```python
from build123d import *

# Parameters (mm, degrees)
BOSS_EXTRUDE3_DEPTH = 90
SKETCH3_W           = 60
SKETCH3_H           = 60
BOSS_EXTRUDE4_DEPTH = 10
BOSS_EXTRUDE5_DEPTH = 24
CUT_EXTRUDE1_REACH  = 101.499
SKETCH6_R           = 2
CUT_EXTRUDE2_REACH  = 101.499
SKETCH7_R           = 2
CUT_EXTRUDE3_REACH  = 101.499
SKETCH9_R           = 2
CUT_EXTRUDE4_REACH  = 101.499
SKETCH10_R          = 2


with BuildPart() as part:
    # Sketch1 → Boss-Extrude3 (new body)
    with BuildSketch(Plane(origin=(0, 0, 0), x_dir=(1, 0, 0), z_dir=(0, 1, 0))):
        with BuildLine():
            Line((-20, 30), (20, 30))
            ThreePointArc((20, 30), (22.928932188, 22.928932188), (30, 20))
            Line((30, 20), (30, -20))
            ThreePointArc((30, -20), (22.928932188, -22.928932188), (20, -30))
            Line((20, -30), (-20, -30))
            ThreePointArc((-20, -30), (-22.928932188, -22.928932188), (-30, -20))
            Line((-30, -20), (-30, 20))
            ThreePointArc((-30, 20), (-22.928932188, 22.928932188), (-20, 30))
        make_face()
    extrude(amount=BOSS_EXTRUDE3_DEPTH)

    # Sketch3 → Boss-Extrude4 (add)
    with BuildSketch(Plane(origin=(0, 90, 0), x_dir=(1, 0, 0), z_dir=(0, 1, 0))):
        Rectangle(SKETCH3_W, SKETCH3_H)
    extrude(amount=BOSS_EXTRUDE4_DEPTH)

    # Sketch4 → Boss-Extrude5 (add)
    with BuildSketch(Plane(origin=(0, 100, 0), x_dir=(1, 0, 0), z_dir=(0, 1, 0))):
        with BuildLine():
            Line((-3.25, 2.331844763), (3.25, 2.331844763))
            ThreePointArc((3.25, 2.331844763), (0, -4), (-3.25, 2.331844763))
        make_face()
    extrude(amount=BOSS_EXTRUDE5_DEPTH)

    # Sketch6 → Cut-Extrude1 (cut, up to next)
    with BuildSketch(Plane.XZ.offset(-90), mode=Mode.PRIVATE) as cut_extrude1_sk1:
        with Locations(Location((-26.408079858, -26.352396966, 0), (0, 0, 270))):
            Circle(SKETCH6_R)
    cut_extrude1_tool1 = extrude(cut_extrude1_sk1.sketch, amount=-CUT_EXTRUDE1_REACH, mode=Mode.PRIVATE) & part.part
    add(cut_extrude1_tool1.solids().sort_by_distance((-26.40808, 90, -26.352397))[0], mode=Mode.SUBTRACT)

    # Sketch7 → Cut-Extrude2 (cut, up to next)
    with BuildSketch(Plane.XZ.offset(-90), mode=Mode.PRIVATE) as cut_extrude2_sk1:
        with Locations(Location((-26.47347716, 26.455477937, 0), (0, 0, 270))):
            Circle(SKETCH7_R)
    cut_extrude2_tool1 = extrude(cut_extrude2_sk1.sketch, amount=-CUT_EXTRUDE2_REACH, mode=Mode.PRIVATE) & part.part
    add(cut_extrude2_tool1.solids().sort_by_distance((-26.473477, 90, 26.455478))[0], mode=Mode.SUBTRACT)

    # Sketch9 → Cut-Extrude3 (cut, up to next)
    with BuildSketch(Plane.XZ.offset(-90), mode=Mode.PRIVATE) as cut_extrude3_sk1:
        with Locations(Location((26.496913455, 26.496913455, 0), (0, 0, 270))):
            Circle(SKETCH9_R)
    cut_extrude3_tool1 = extrude(cut_extrude3_sk1.sketch, amount=-CUT_EXTRUDE3_REACH, mode=Mode.PRIVATE) & part.part
    add(cut_extrude3_tool1.solids().sort_by_distance((26.496913, 90, 26.496913))[0], mode=Mode.SUBTRACT)

    # Sketch10 → Cut-Extrude4 (cut, up to next)
    with BuildSketch(Plane.XZ.offset(-90), mode=Mode.PRIVATE) as cut_extrude4_sk1:
        with Locations(Location((26.464466094, -26.464466094, 0), (0, 0, 270))):
            Circle(SKETCH10_R)
    cut_extrude4_tool1 = extrude(cut_extrude4_sk1.sketch, amount=-CUT_EXTRUDE4_REACH, mode=Mode.PRIVATE) & part.part
    add(cut_extrude4_tool1.solids().sort_by_distance((26.464466, 90, -26.464466))[0], mode=Mode.SUBTRACT)


solid = part.part
```
The model under review builds one solid part; all positions refer to its coordinate system, in mm. A direction names the side the tool comes from. Give positions to 0.01 mm unless a question says otherwise; leave off trailing zeros. Write each loop counter-clockwise with the first axis right and the second up, starting at its lowest first coordinate (ties: lowest second). Pieces come first, ordered by that corner, then holes.
(1) Consider section C-C, the plane x = 6.5. Give the boundary of the cut face in (y, z), and give its area (3 significant figures).
(2) The part is to be moulded in two halves that separate along Z. For faces 6 (the flat face through (0, 49, 30)), 7 (the cylindrical face through (25.698, 94.93, -28.312)), 8 (the flat face through (-30, 49, 0)), say which applies: released by +Z, released by -Z, zero draft, split by the parting line, or undercut.
(3) For P1, Ø6, axis at x = 0, z = 13, coming from the +Y side; P2, Ø5, axis at x = -26.47, z = 26.46, coming from the -Y side; P3, Ø1.5, axis at x = -24, y = 39, coming from the +Z side, all flat-tipped, find the tip position at first contact; note any pin that passes through.
(4) Tool access review of faces 1 (the cylindrical face through (-23.01, 44.37, -22.85)), 2 (the flat face through (24, 90, -26)), 3 (the flat face through (-26, 90, 24)), 4 (the cylindrical face through (0, 112, 4)), 5 (the flat face through (0, 112, -2.332)): name each direction out of +Z, -Z, +X, -X, +Y, -Y from which nothing blocks a thin tool from reaching the whole face with its end or side.
(5) Consider section D-D, the plane y = 102.5. Give the boundary of the cut face in (x, z).
(6) Consider section A-A, the plane y = 17.5. Give the boundary of the cut face in (x, z).
(7) To check wall thickness, follow L1, parallel to Y at x = -20, z = -20.5; L2, parallel to Y at x = 25.5, z = 24.5; L3, parallel to X at y = 60.5, z = -27. State the ranges of each line that lie inside material, in increasing order.
(8) Consider section B-B, the plane z = 0. Give the boundary of the cut face in (x, y).
Returned:
1. outline: (0, -30) - (100, -30) - (100, 30) - (0, 30) - close
1. area: 6,000 mm2
2. face 6: released by +Z
2. face 7: undercut
2. face 8: zero draft
3. P1: stops at y = 100
3. P2: stops at y = 90
3. P3: stops at z = 22.62
4. face 1: -Z, -X, -Y
4. face 2: -Z, +X, -Y
4. face 3: +Z, -X, -Y
4. face 4: +Y
4. face 5: -Z, +X, -X, +Y
5. outline: (-3.25, -2.33) - (3.25, -2.33) arc R4 ccw (long way) to start
6. outline: (-30, -20) arc R10 cw to (-20, -30) - (20, -30) arc R10 cw to (30, -20) - (30, 20) arc R10 cw to (20, 30) - (-20, 30) arc R10 cw to (-30, 20) - close
7. L1: y = 0 to 100
7. L2: y = 90 to 100
7. L3: x = -20.46 to 20.46
8. outline: (-30, 0) - (30, 0) - (30, 100) - (4, 100) - (4, 124) - (-4, 124) - (-4, 100) - (-30, 100) - close
